The figure shows three views and two pictorial views of one solid part (mm, origin at its lowest corner). Answer the questions. Coordinates: 2 decimals unless noted, no trailing zeros. Order: outer loops, then holes, each group sorted by start corner. A loop starts at its lowest first (then second) coordinate and runs counter-clockwise, first axis right, second up. Notation, with made-up numbers: M 76.25,-29 L 94.25,-29 A36 cw 94.25,6 Z; hole C 86.25,52.5 d5. An arc over 180 degrees is marked long. Answer in a Markdown table with one row per item. Add a question column.
Item 1: The part is cut by section A-A (x = 105). Write down the section's boundary in (y, z).
Item 2: The part is cut by section B-B (z = 61). Write down the section's boundary in (x, y).
Item 3: Consider line 1 (Z direction, x = 149.5, y = 1.45); line 2 (X direction, y = 1.1, z = 19.5); line 3 (X direction, y = 1.4, z = 82.5). Determine where each line is inside the solid, lowest interval first. Write a range as from..to.
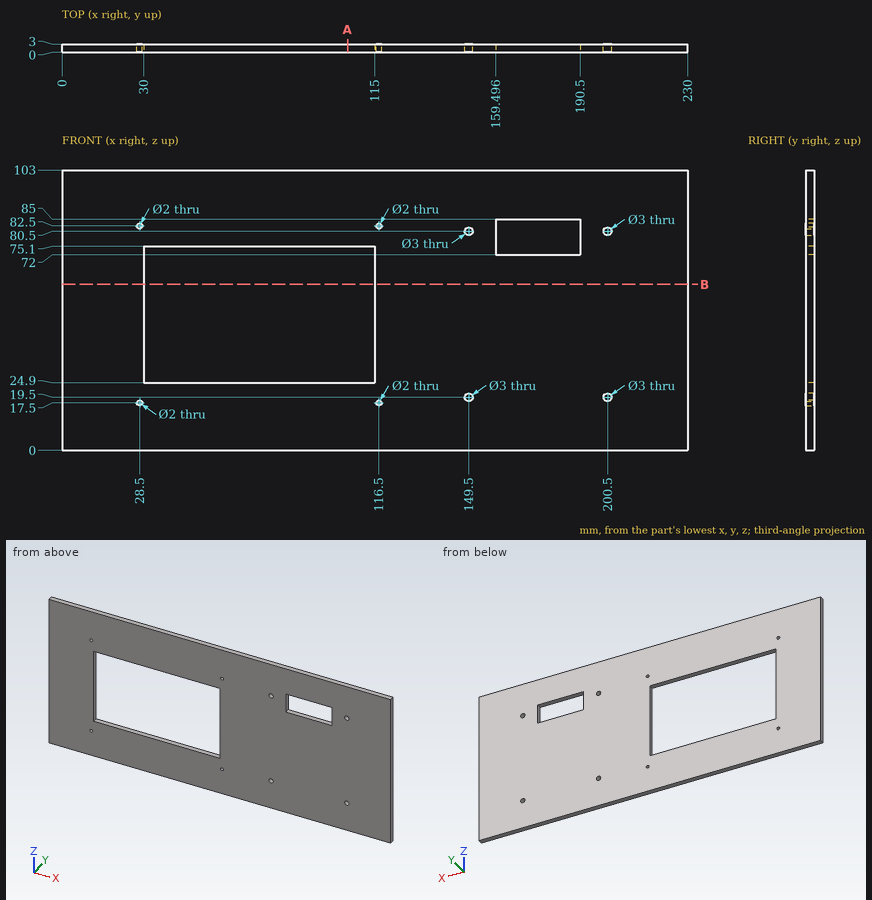
Reply:
| question | item | result |
|---|---|---|
| 1 | outline | M 0,0 L 3,0 L 3,24.9 L 0,24.9 Z; M 0,75.1 L 3,75.1 L 3,103 L 0,103 Z |
| 2 | outline | M 0,0 L 30,0 L 30,3 L 0,3 Z; M 115,0 L 230,0 L 230,3 L 115,3 Z |
| 3 | line 1 | z = 0..18, 21..79, 82..103 |
| 3 | line 2 | x = 0..148, 151..199, 202..230 |
| 3 | line 3 | x = 0..27.5, 29.5..115.5, 117.5..159.5, 190.5..230 |
